Input: part model. Units: mm. Frame: model coordinates. A direction names the side the tool comes from. Coordinates: 2 decimals unless noted, no trailing zeros. Write each loop counter-clockwise with the first axis right and the second up, starting at its lowest first coordinate (ties: lowest second). Pieces come first, ordered by that corner, then holes.
from build123d import *

# Parameters (mm, degrees)
F0_R     = 8
F0_R_2   = 4.125
F1_DEPTH = 13.5
F2_R     = 4.6
F3_DEPTH = 12.5
F4_R     = 6.125
F5_DEPTH = 4.5
F6_SIZE  = 0.5


with BuildPart() as f1:
    # F0 (on Top) → F1 (new body)
    with BuildSketch(Plane.XY):
        Circle(F0_R)
        Circle(F0_R_2, mode=Mode.SUBTRACT)
    extrude(amount=F1_DEPTH)

    # F2 (on Top) → F3 (cut)
    with BuildSketch(Plane.XY):
        Circle(F2_R)
    extrude(amount=F3_DEPTH, mode=Mode.SUBTRACT)

    # F4 (on Top) → F5 (cut)
    with BuildSketch(Plane.XY):
        Circle(F4_R)
    extrude(amount=F5_DEPTH, mode=Mode.SUBTRACT)

    # F6
    f6_edges = [f1.edges().sort_by_distance(p)[0] for p in [
        (-4.125, 0, 13.5),
    ]]
    chamfer(f6_edges, length=F6_SIZE)


solid = f1.part
Item 1: Pin query (flat end, axial travel): pin 1 Ø4 at (x, z) = (-5.5, 4.5) entering from -Y; pin 2 Ø7.5 at (x, y) = (0, 0) entering from -Z; pin 3 Ø5 at (y, z) = (5, 9.5) entering from -X; pin 4 Ø1 at (x, y) = (4, 0) entering from -Z. Return the tip coordinate at first contact, or that it passes through.
Item 2: Section query C-C, the plane z = 5. Return loops of the section in (x, y), then the cut area to 3 significant figures.
Item 3: Section query D-D, the plane z = 1.5. Return loops of the section in (x, y) (3 decimals).
Item 4: Material intervals for line 1 (Y direction, x = 0, z = 12.9) (3 decimals); line 2 (Y direction, x = 0, z = 9.5); line 3 (X direction, y = -3, z = 1.75), sorted ascending.
Item 5: Section query B-B, the plane y = 5. Return loops of the section in (x, z) (3 decimals).
Item 6: Section query A-A, the plane x = 0. Return loops of the section in (y, z) (3 decimals).
Item 7: Access query for faces 4 (the face through (1, 5, 4.5)), 5 (the face through (-2, -6, 0)). Directions: +Z, -Z, +X, -X, +Y, -Y. A direction counts if a zero-diameter tool reaches every point of the face in a straight line with its end or side. Return the directions, or none.
Item 8: Pull-direction query (X, two-part tool) for faces 1 (the face through (-3.65, -2.8, 8.44)), 2 (the face through (3.4, -3.4, 13.5)), 3 (the face through (-1.73, -7.81, 6.66)); classes: released by +X, released by -X, zero draft, split by the parting line, or undercut.
The answers:
1. pin 1: stops at y = -7.19
1. pin 2: passes through
1. pin 3: stops at x = -7.6
1. pin 4: stops at z = 12.5
2. outline: circle Ø16 at (0, 0); hole circle Ø9.2 at (0, 0)
2. area: 135 mm2
3. outline: circle Ø16 at (0, 0); hole circle Ø12.25 at (0, 0)
4. line 1: y = -8 to -4.125, 4.125 to 8
4. line 2: y = -8 to -4.6, 4.6 to 8
4. line 3: x = -7.42 to -5.34, 5.34 to 7.42
5. outline: (-6.245, 0) - (-3.538, 0) - (-3.538, 4.5) - (3.538, 4.5) - (3.538, 0) - (6.245, 0) - (6.245, 13.5) - (-6.245, 13.5) - close
6. outline: (-8, 0) - (-6.125, 0) - (-6.125, 4.5) - (-4.6, 4.5) - (-4.6, 12.5) - (-4.125, 12.5) - (-4.125, 13) - (-4.625, 13.5) - (-8, 13.5) - close; (4.125, 12.5) - (4.6, 12.5) - (4.6, 4.5) - (6.125, 4.5) - (6.125, 0) - (8, 0) - (8, 13.5) - (4.625, 13.5) - (4.125, 13) - close
7. face 4: -Z
7. face 5: -Z, +X, -X, +Y, -Y
8. face 1: undercut
8. face 2: zero draft
8. face 3: split by the parting line
